Input: part model. Units: mm. Frame: model coordinates. A direction names the side the tool comes from. Coordinates: 2 decimals unless noted, no trailing zeros. Write each loop counter-clockwise with the first axis right and the second up, starting at its lowest first coordinate (ties: lowest second). Pieces come first, ordered by that corner, then holes. Notation, with made-up numbers: (-16.5, 12) -> (-12.5, 12) arc R13 cw to (-12.5, 19) -> close; hole circle Ø4 at (14.25, 82). An arc over 180 degrees is marked (long way). Use one line per item in the form item = value. Start each with the question number.
(1) Cut plane A-A on x = -44. Return the cut outline in (y, z).
(2) Cut plane B-B on z = 19. Return the cut outline in (x, y).
(3) Ray query, line 1 along Z through (x, y) = (6.35, -3.5); line 2 along X through (y, z) = (-6.75, -31); line 3 along X through (y, z) = (-6.5, 1.5). Return the intervals inside material, ascending.
(4) Set-up query: faces 4 (the face through (76.708, -5, 17)), 5 (the face through (16.698, -4.884, 40.954)), 6 (the face through (-80, -5, -6.414)), 7 (the face through (76.708, -5, 51)). Return all of +Z, -Z, +X, -X, +Y, -Y with unobstructed straight access to the full face (end or side cutting, diameter ignored); none if empty.
(5) Pull-direction query (X, two-part tool) for faces 1 (the face through (80, -5, 30.162)), 2 (the face through (-20.066, -5, 51)), 3 (the face through (-76.708, -5, -20)); classes: released by +X, released by -X, zero draft, split by the parting line, or undercut.
(6) First-contact query: pin 1 (3 mm diameter, centred on y = -4, z = 19.5, fed in from -X); pin 2 (2.5 mm diameter, centred on x = -80.772, z = 0, fed in from -Y). Flat tips, straight axial feed; report the tip coordinate or a pass-through.
```python
from build123d import *

# Parameters (mm, degrees)
F1_DEPTH = 9.906
F2_SIZE  = 1.905
F4_D     = 2.7051
F4_DEPTH = 8.73125
F4_TIP   = 0.8126940303
F6_D     = 3.2639


with BuildPart() as f1:
    # F0 (on Front) → F1 (new body)
    with BuildSketch(Plane.XZ):
        with BuildLine():
            ThreePointArc((-85.09, -51.7525), (-83.7880896424, -54.8955896424), (-80.645, -56.1975))
            Line((-80.645, -56.1975), (80.645, -56.1975))
            ThreePointArc((80.645, -56.1975), (83.7880896424, -54.8955896424), (85.09, -51.7525))
            Line((85.09, -51.7525), (85.09, -34.8615))
            Line((85.09, -34.8615), (76.708, -34.8615))
            Line((76.708, -34.8615), (76.708, -6.4135))
            Line((76.708, -6.4135), (85.09, -6.4135))
            Line((85.09, -6.4135), (85.09, 4.2545))
            Line((85.09, 4.2545), (76.708, 4.2545))
            Line((76.708, 4.2545), (76.708, 30.1625))
            Line((76.708, 30.1625), (85.09, 30.1625))
            Line((85.09, 30.1625), (85.09, 51.7525))
            ThreePointArc((85.09, 51.7525), (83.7880896424, 54.8955896424), (80.645, 56.1975))
            Line((80.645, 56.1975), (76.708, 56.1975))
            Line((76.708, 56.1975), (76.708, 47.8155))
            Line((76.708, 47.8155), (65.278, 47.8155))
            Line((65.278, 47.8155), (65.278, 56.1975))
            Line((65.278, 56.1975), (56.896, 56.1975))
            Line((56.896, 56.1975), (56.896, 47.8155))
            Line((56.896, 47.8155), (20.066, 47.8155))
            Line((20.066, 47.8155), (20.066, 56.1975))
            Line((20.066, 56.1975), (-20.066, 56.1975))
            Line((-20.066, 56.1975), (-20.066, 47.8155))
            Line((-20.066, 47.8155), (-56.896, 47.8155))
            Line((-56.896, 47.8155), (-56.896, 56.1975))
            Line((-56.896, 56.1975), (-65.278, 56.1975))
            Line((-65.278, 56.1975), (-65.278, 47.8155))
            Line((-65.278, 47.8155), (-76.708, 47.8155))
            Line((-76.708, 47.8155), (-76.708, 56.1975))
            Line((-76.708, 56.1975), (-80.645, 56.1975))
            ThreePointArc((-80.645, 56.1975), (-83.7880896424, 54.8955896424), (-85.09, 51.7525))
            Line((-85.09, 51.7525), (-85.09, 30.1625))
            Line((-85.09, 30.1625), (-76.708, 30.1625))
            Line((-76.708, 30.1625), (-76.708, 4.2545))
            Line((-76.708, 4.2545), (-85.09, 4.2545))
            Line((-85.09, 4.2545), (-85.09, -6.4135))
            Line((-85.09, -6.4135), (-76.708, -6.4135))
            Line((-76.708, -6.4135), (-76.708, -34.8615))
            Line((-76.708, -34.8615), (-85.09, -34.8615))
            Line((-85.09, -34.8615), (-85.09, -51.7525))
        make_face()
        with BuildLine():
            ThreePointArc((-15.4305, -37.846), (-16.7324103576, -40.9890896424), (-19.8755, -42.291))
            Line((-19.8755, -42.291), (-67.2465, -42.291))
            ThreePointArc((-67.2465, -42.291), (-70.3895896424, -40.9890896424), (-71.6915, -37.846))
            Line((-71.6915, -37.846), (-71.6915, 37.846))
            ThreePointArc((-71.6915, 37.846), (-70.3895896424, 40.9890896424), (-67.2465, 42.291))
            Line((-67.2465, 42.291), (-19.8755, 42.291))
            ThreePointArc((-19.8755, 42.291), (-16.7324103576, 40.9890896424), (-15.4305, 37.846))
            Line((-15.4305, 37.846), (-15.4305, -37.846))
        make_face(mode=Mode.SUBTRACT)
        with BuildLine():
            Line((71.6915, 37.846), (71.6915, -37.846))
            ThreePointArc((71.6915, -37.846), (70.3895896424, -40.9890896424), (67.2465, -42.291))
            Line((67.2465, -42.291), (19.8755, -42.291))
            ThreePointArc((19.8755, -42.291), (16.7324103576, -40.9890896424), (15.4305, -37.846))
            Line((15.4305, -37.846), (15.4305, 37.846))
            ThreePointArc((15.4305, 37.846), (16.7324103576, 40.9890896424), (19.8755, 42.291))
            Line((19.8755, 42.291), (67.2465, 42.291))
            ThreePointArc((67.2465, 42.291), (70.3895896424, 40.9890896424), (71.6915, 37.846))
        make_face(mode=Mode.SUBTRACT)
    extrude(amount=F1_DEPTH)

    # F2
    f2_edges = [f1.edges().sort_by_distance(p)[0] for p in [
        (-85.09, -4.953, -34.8615),
        (-85.09, -4.953, -6.4135),
        (-85.09, -4.953, 4.2545),
        (-85.09, -4.953, 30.1625),
        (-76.708, -4.953, 56.1975),
        (-65.278, -4.953, 56.1975),
        (-56.896, -4.953, 56.1975),
        (-20.066, -4.953, 56.1975),
        (20.066, -4.953, 56.1975),
        (65.278, -4.953, 56.1975),
        (56.896, -4.953, 56.1975),
        (76.708, -4.953, 56.1975),
        (85.09, -4.953, 30.1625),
        (85.09, -4.953, 4.2545),
        (85.09, -4.953, -6.4135),
        (85.09, -4.953, -34.8615),
    ]]
    chamfer(f2_edges, length=F2_SIZE)

    # F4
    with Locations(Plane.XZ.offset(9.906)):
        with Locations((-80.772, 51.6255), (-80.772, 0), (-80.772, -51.6255), (-6.35, -51.6255), (-6.35, 0), (-6.35, 51.6255), (6.35, 51.6255), (6.35, 0), (6.35, -51.6255), (80.772, -51.6255), (80.772, 0), (80.772, 51.6255)):
            Hole(F4_D / 2, depth=F4_DEPTH)
            with Locations((0, 0, -(F4_DEPTH + F4_TIP / 2))):  # 118° drill point
                Cone(0, F4_D / 2, F4_TIP, mode=Mode.SUBTRACT)

    # F6 (through all)
    with Locations(Plane.XZ.offset(9.906)):
        with Locations((-81.026, 34.6075), (-62.992, 52.1335), (-81.026, -39.4335), (-62.992, -52.1335), (-17.526, 52.1335), (-17.526, -52.1335), (0, 6.4135), (17.526, -52.1335), (62.992, -52.1335), (81.026, -39.4335), (81.026, 34.6075), (62.992, 52.1335), (17.526, 52.1335)):
            Hole(F6_D / 2)


solid = f1.part
```
Values:
q1.outline = (-9.91, -56.2) -> (0, -56.2) -> (0, -42.29) -> (-9.91, -42.29) -> close; (-9.91, 42.29) -> (0, 42.29) -> (0, 47.82) -> (-9.91, 47.82) -> close
q2.outline = (-76.71, -9.91) -> (-71.69, -9.91) -> (-71.69, 0) -> (-76.71, 0) -> close; (-15.43, -9.91) -> (15.43, -9.91) -> (15.43, 0) -> (-15.43, 0) -> close; (71.69, -9.91) -> (76.71, -9.91) -> (76.71, 0) -> (71.69, 0) -> close
q3.line_1 = -56.2 to -52.98, -50.27 to -1.35, 1.35 to 50.27, 52.98 to 56.2
q3.line_2 = -76.71 to -71.69, -15.43 to 15.43, 71.69 to 76.71
q3.line_3 = -85.09 to -71.69, -15.43 to 15.43, 71.69 to 85.09
q4.face_4 = +X, +Y, -Y
q4.face_5 = +Y, -Y
q4.face_6 = -X, +Y, -Y
q4.face_7 = +Z, +Y, -Y
q5.face_1 = zero draft
q5.face_2 = undercut
q5.face_3 = released by -X
q6.pin_1 = -76.71
q6.pin_2 = -1.11
